Geometry check sheet. Reference: the model listing, model coordinates, mm. A direction names the side the tool comes from. Give positions to 0.01 mm unless a question says otherwise; leave off trailing zeros. Order: outer loops, then holes, each group sorted by start corner. A loop starts at its lowest first (then second) coordinate and runs counter-clockwise, first axis right, second up. Notation, with made-up numbers: M 32.25,-35.75 L 63.25,-35.75 A18 ccw 63.25,-17.75 Z; hole C 82,-15 d5. An arc over 180 degrees is marked long. Answer as CSV lines item,"result".
Solid Edge part; units mm, degrees
sketch "Sketch1" plane through (0, 0, 0) normal (0, 0, 1) x (1, 0, 0)
  line L0 (10, -50) -> (-10, -50)
  line L1 (-10, -50) -> (-10, 50)
  line L2 (-10, 50) -> (10, 50)
  line L3 (10, 50) -> (10, -50)
  dimension "D1" = 10
  dimension "D2" = 10
extrude "Ajout_matière_1" add sketch "Sketch1" along normal blind 15
sketch "Sketch2" plane through (0, 0, 15) normal (0, 0, 1) x (1, 0, 0)
  line L0 (6.4998, -46.5) -> (-6.4998, -46.5)
  line L1 (-6.4998, -46.5) -> (-6.4998, 46.5)
  line L2 (-6.4998, 46.5) -> (6.4998, 46.5)
  line L3 (6.4998, 46.5) -> (6.4998, -46.5)
extrude "Enlèvement_matière_1" cut sketch "Sketch2" against normal blind 8.2123
sketch "Sketch3" plane through (10, 0, 7.5) normal (1, 0, 0) x (0, 0, -1)
  circle A0 centre (5, 0) radius 2
  dimension "D1" = 5
extrude "Cutout1" cut sketch "Sketch3" against normal through all
sketch "Sketch4" plane through (0, 0, 0) normal (0, 0, -1) x (1, 0, 0)
  line L0 (-10, -50) -> (10, -50)
  line L1 (10, -50) -> (10, 50)
  line L2 (10, 50) -> (-10, 50)
  line L3 (-10, 50) -> (-10, -50)
extrude "Ajout_matière_2" add sketch "Sketch4" along normal blind 4.5
sketch "Sketch5" plane through (0, 0, -4.5) normal (0, 0, -1) x (0, -1, 0)
  line L0 (20, -3.843) -> (5, -3.843)
  line L1 (5, -3.843) -> (5, 4.157)
  line L2 (5, 4.157) -> (20, 4.157)
  line L3 (20, 4.157) -> (20, -3.843)
  dimension "D1" = 5
  dimension "D2" = 20
extrude "Cutout2" cut sketch "Sketch5" against normal through all
properties material "Acier S235"
(1) Material ranges on line 1 (Y direction, x = -1.5, z = 2.5); line 2 (X direction, y = -17.5, z = 4.25); line 3 (X direction, y = 40, z = 8.25), recorded low to high.
The answers:
line 1,"y = -50 to -20, -5 to -2, 2 to 50"
line 2,"x = -10 to -4.16, 3.84 to 10"
line 3,"x = -10 to -6.5, 6.5 to 10"
(2) Draft check along Y on faces 4 (the face through (0, 1, 6.788)), 5 (the face through (0, 1, -4.5)), 6 (the face through (0, 50, 5)). Enter one of: +Y half, -Y half, draft (parallel to the pull), parting line (faces both ways), or undercut.
The answers:
face 4,"undercut"
face 5,"draft"
face 6,"+Y half"
(3) Section check C-C on x = 1. Enter the section's corners in (y, z).
The answers:
outline,"M -50,-4.5 L -20,-4.5 L -20,6.79 L -46.5,6.79 L -46.5,15 L -50,15 Z; M -5,-4.5 L 50,-4.5 L 50,15 L 46.5,15 L 46.5,6.79 L -5,6.79 Z; hole C 0,2.5 d4"
(4) Section check A-A on y = 0. Enter the section's corners in (x, z).
The answers:
outline,"M -10,-4.5 L 10,-4.5 L 10,0.5 L -10,0.5 Z; M -10,4.5 L 10,4.5 L 10,15 L 6.5,15 L 6.5,6.79 L -6.5,6.79 L -6.5,15 L -10,15 Z"
(5) Section check D-D on z = 10.25. Enter the section's corners in (x, y), then the cut area to 3 significant figures.
The answers:
outline,"M -10,-50 L 10,-50 L 10,50 L -10,50 Z; hole M -6.5,-46.5 L 6.5,-46.5 L 6.5,46.5 L -6.5,46.5 Z"
area,"791 mm2"
(6) Section check B-B on z = 2.5. Enter the section's corners in (x, y), then the cut area to 3 significant figures.
The answers:
outline,"M -10,-50 L 10,-50 L 10,-2 L -10,-2 Z; M -10,2 L 10,2 L 10,50 L -10,50 Z; hole M -4.16,-20 L 3.84,-20 L 3.84,-5 L -4.16,-5 Z"
area,"1,800 mm2"
(7) Tool access check on faces 1 (the face through (6.5, 1, 11)), 2 (the face through (0, -5, 1)), 3 (the face through (10, 1, 5)). Record the directions out of +Z, -Z, +X, -X, +Y, -Y that give a thin tool (end or side, any length) a straight path to the whole face; none if there is none.
The answers:
face 1,"+Z"
face 2,"+Z, -Z"
face 3,"+Z, -Z, +X, +Y, -Y"
